Check sheet for the drawn part. Datum: minimum x, y, z corner. Units: mm. A direction names the side the tool comes from. Give positions to 0.01 mm unless a question says otherwise; leave off trailing zeros. Write each loop counter-clockwise with the first axis right and the second up, starting at its lowest first coordinate (ties: lowest second). Pieces come first, ordered by that corner, then holes.
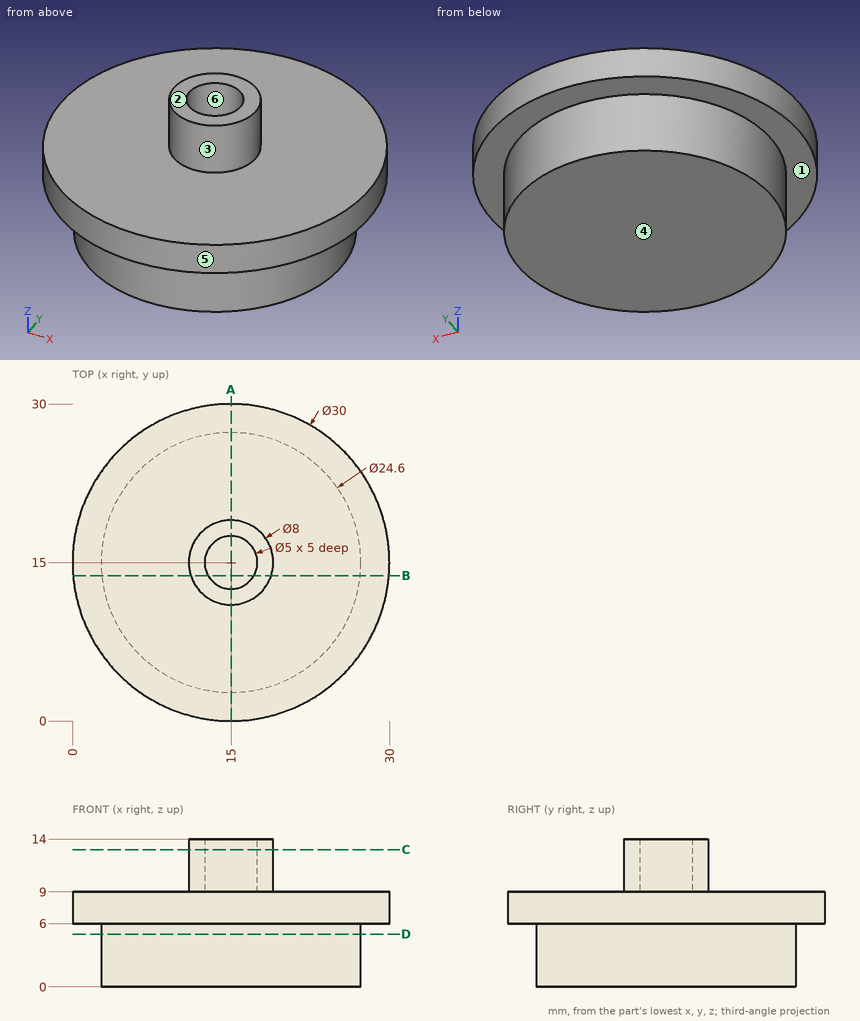
1) Sectioned sample at D-D on z = 5. Record the boundary of the cut face in (x, y), then the cut area to 3 significant figures.
2) Sectioned sample at A-A on x = 15. Record the boundary of the cut face in (y, z), then the cut area to 3 significant figures.
3) Sectioned sample at B-B on y = 13.75. Record the boundary of the cut face in (x, z).
4) Scan lines: L1, parallel to Y at x = 15, z = 10.9; L2, parallel to Z at x = 19.75, y = 15.5; L3, parallel to Z at x = 3, y = 10. Record each from-to range of solid material in increasing order.
5) Access from +Z, -Z, +X, -X, +Y, -Y to the whole of each face (thin tool, end or side, straight path). Record for the marked faces 1, 2 and 3.
6) Gauge pin test, flat ends, axial feed: pin 1 (2 mm diameter, centred on y = 8, z = 9, fed in from -X); pin 2 (1.5 mm diameter, centred on y = 13.5, z = 9.5, fed in from -X); pin 3 (2 mm diameter, centred on x = 13, y = 23, fed in from +Z). Record the tip position at first contact, or that the pin passes through.
7) Sectioned sample at C-C on z = 13. Record the boundary of the cut face in (x, y).
8) Draft check along Y on the marked faces 4, 5 and 6. Enter one of: +Y half, -Y half, draft (parallel to the pull), parting line (faces both ways), or undercut.
Answers below:
1. outline: circle Ø24.6 at (15, 15)
1. area: 475 mm2
2. outline: (0, 6) - (2.7, 6) - (2.7, 0) - (27.3, 0) - (27.3, 6) - (30, 6) - (30, 9) - (19, 9) - (19, 14) - (17.5, 14) - (17.5, 9) - (12.5, 9) - (12.5, 14) - (11, 14) - (11, 9) - (0, 9) - close
2. area: 253 mm2
3. outline: (0.05, 6) - (2.76, 6) - (2.76, 0) - (27.24, 0) - (27.24, 6) - (29.95, 6) - (29.95, 9) - (18.8, 9) - (18.8, 14) - (17.17, 14) - (17.17, 9) - (12.83, 9) - (12.83, 14) - (11.2, 14) - (11.2, 9) - (0.05, 9) - close
4. L1: y = 11 to 12.5, 17.5 to 19
4. L2: z = 0 to 9
4. L3: z = 6 to 9
5. face 1: -Z
5. face 2: +Z, +X, -X, +Y, -Y
5. face 3: +Z
6. pin 1: stops at x = 1.25
6. pin 2: stops at x = 0.03
6. pin 3: stops at z = 9
7. outline: circle Ø8 at (15, 15); hole circle Ø5 at (15, 15)
8. face 4: draft
8. face 5: parting line
8. face 6: undercut
